Design review of the part built by this model. Coordinates are the model's own, in mm. A direction names the side the tool comes from. Give positions to 0.01 mm unless a question says otherwise; leave off trailing zeros. Loops run counter-clockwise (first coordinate to the right, second up) from the corner with the lowest first, then second, coordinate; pieces in that order, holes last. Notation, with made-up numbers: M 10.25,53 L 41.25,53 A10 ccw 41.25,68 Z; hole C 87.25,-13 d9. An arc over 180 degrees is marked long. Use CSV: the item, a comma, the result in double quotes.
from build123d import *

# Parameters (mm, degrees)
F0_R             = 14.605
F1_DEPTH         = 9.017
F2_R             = 6.35
F3_DEPTH         = 27.94
F4_R             = 5.334
F5_DEPTH         = 40.64
F6_R             = 8.255
F7_DEPTH         = 2.3
F8_R             = 5.06
F9_DEPTH         = 4.1
F11_D            = 3.1
F13_DEPTH        = 40.64
F13_COPIES_COUNT = 6
F14_R            = 0.508


# Not quite as in the source:
# - a pattern or mirror of a feature is missing from the dataset's text; its kind, count and spacing are read off the source's solid


with BuildPart() as f1:
    # F0 (on Top) → F1 (new body)
    with BuildSketch(Plane.XY):
        Circle(F0_R)
    extrude(amount=F1_DEPTH)

    # F2 (on face) → F3 (join)
    with BuildSketch(Plane.XY.offset(9.017)):
        Circle(F2_R)
    extrude(amount=F3_DEPTH)

    # F4 (on face) → F5 (join)
    with BuildSketch(Plane.XY.offset(36.957)):
        Circle(F4_R)
    extrude(amount=F5_DEPTH)

    # F6 (on face) → F7 (cut)
    with BuildSketch(Plane(origin=(0, 0, 0), x_dir=(1, 0, 0), z_dir=(0, 0, -1))):
        Circle(F6_R)
    extrude(amount=-F7_DEPTH, mode=Mode.SUBTRACT)

    # F8 (on face) → F9 (cut)
    with BuildSketch(Plane(origin=(0, 0, 0), x_dir=(1, 0, 0), z_dir=(0, 0, -1))):
        Circle(F8_R)
    extrude(amount=-F9_DEPTH, mode=Mode.SUBTRACT)

    # F11 (through all)
    with Locations(Plane.XY.offset(9.017)):
        with Locations((0, -10.05), (-10.05, 0), (0, 10.05), (10.05, 0)):
            Hole(F11_D / 2)

    # F12 (on face) → F13 (join, through all)
    with BuildSketch(Plane.XY.offset(77.597)):
        with BuildLine():
            Line((-1.27, -5.1806038258), (-1.27, -6.1957780109))
            ThreePointArc((-1.27, -6.1957780109), (0, -6.3246), (1.27, -6.1957780109))
            Line((1.27, -6.1957780109), (1.27, -5.1806038258))
            ThreePointArc((1.27, -5.1806038258), (0, -5.334), (-1.27, -5.1806038258))
        make_face()
    f13 = extrude(amount=-F13_DEPTH)

    # F13_copies: F13 ×6 about axis
    f13_copies_axis = Axis((0, 0, 0), (0, 0, 1))
    for i in range(1, F13_COPIES_COUNT):
        add(f13.rotate(f13_copies_axis, i * 360 / F13_COPIES_COUNT))

    # F14
    f14_edges = [f1.edges().sort_by_distance(p)[0] for p in [
        (1.27, -6.195778, 57.277),
        (1.27, -5.180604, 57.277),
        (-1.27, -6.195778, 57.277),
        (-1.27, -5.180604, 57.277),
        (3.851535, -3.690154, 57.277),
        (4.730701, -4.197741, 57.277),
        (6.000701, -1.998037, 57.277),
        (5.121535, -1.49045, 57.277),
        (5.121535, 1.49045, 57.277),
        (6.000701, 1.998037, 57.277),
        (4.730701, 4.197741, 57.277),
        (3.851535, 3.690154, 57.277),
        (1.27, 5.180604, 57.277),
        (1.27, 6.195778, 57.277),
        (-1.27, 6.195778, 57.277),
        (-1.27, 5.180604, 57.277),
        (-3.851535, 3.690154, 57.277),
        (-4.730701, 4.197741, 57.277),
        (-6.000701, 1.998037, 57.277),
        (-5.121535, 1.49045, 57.277),
        (-5.121535, -1.49045, 57.277),
        (-6.000701, -1.998037, 57.277),
        (-4.730701, -4.197741, 57.277),
        (-3.851535, -3.690154, 57.277),
    ]]
    fillet(f14_edges, radius=F14_R)


solid = f1.part
(1) Clearance check with flat-ended pins moving along their axes: P1, Ø6, axis at x = -8, z = 66.5, coming from the -Y side; P2, Ø10, axis at y = 2, z = 44, coming from the -X side; P3, Ø2, axis at y = 1, z = 66.5, coming from the +X side. State where each tip first meets the part, or that it passes through.
A:
P1,"y = -3.87"
P2,"x = -5.88"
P3,"x = 5.83"
(2) Machinability: for faces 4 (the cylindrical face through (-1.38, -6.2, 22.79)), 5 (the flat face through (0, 0, 4.1)), 6 (the cylindrical face through (5.483, 3.152, 57.561)), 7 (the cylindrical face through (-5.334, 0.016, 56.993)), 8 (the cylindrical face through (0.012, 6.325, 57.561)), which of the approach directions +Z, -Z, +X, -X, +Y, -Y give a long, thin tool a straight path to every point of the face, cutting with its end or side? Answer none if there is none.
A:
face 4,"+Z"
face 5,"-Z"
face 6,"+Z, +X, +Y"
face 7,"+Z, -X"
face 8,"+Z, +Y"
(3) We need section B-B on x = 0. State the section outline as (y, z) points (3 decimals), then the cut area to 3 significant figures.
A:
outline,"M -14.605,0 L -11.6,0 L -11.6,9.017 L -14.605,9.017 Z; M -8.5,0 L -8.255,0 L -8.255,2.3 L -5.06,2.3 L -5.06,4.1 L 5.06,4.1 L 5.06,2.3 L 8.255,2.3 L 8.255,0 L 8.5,0 L 8.5,9.017 L 6.35,9.017 L 6.35,36.957 L 6.325,36.957 L 6.325,77.597 L -6.325,77.597 L -6.325,36.957 L -6.35,36.957 L -6.35,9.017 L -8.5,9.017 Z; M 11.6,0 L 14.605,0 L 14.605,9.017 L 11.6,9.017 Z"
area,"1,020 mm²"
(4) We need section C-C on y = 10.05. State the section outline as (x, z) points, then the cut area to 3 significant figures.
A:
outline,"M -10.6,0 L -1.55,0 L -1.55,9.02 L -10.6,9.02 Z; M 1.55,0 L 10.6,0 L 10.6,9.02 L 1.55,9.02 Z"
area,"163 mm²"
(5) The part is to be moulded in two halves that separate along Y. For faces 1 (the cylindrical face through (-0.012, -6.325, 57.561)), 2 (the cylindrical face through (2.7, 4.6, 57)), 3 (the cylindrical face through (4.674, 1.938, 3.187)), say which applies: released by +Y, released by -Y, zero draft, split by the parting line, or undercut.
A:
face 1,"released by -Y"
face 2,"released by +Y"
face 3,"undercut"
(6) Wall thickness on line 1 along Y through (x, z) = (0, 3.75) (3 decimals); line 2 along Z through (x, y) = (-10, -5.25); line 3 along Z through (x, y) = (-1.75, -2.5): over which ranges is each line inside the solid? List them lowest first. Write a range as [from, to].
A:
line 1,"[-14.605, -11.6], [-8.5, -5.06], [5.06, 8.5], [11.6, 14.605]"
line 2,"[0, 9.02]"
line 3,"[4.1, 77.6]"
(7) We need section A-A on y = 0. State the section outline as (x, z) points (3 decimals).
A:
outline,"M -14.605,0 L -11.6,0 L -11.6,9.017 L -14.605,9.017 Z; M -8.5,0 L -8.255,0 L -8.255,2.3 L -5.06,2.3 L -5.06,4.1 L 5.06,4.1 L 5.06,2.3 L 8.255,2.3 L 8.255,0 L 8.5,0 L 8.5,9.017 L 6.35,9.017 L 6.35,36.957 L 5.334,36.957 L 5.334,77.597 L -5.334,77.597 L -5.334,36.957 L -6.35,36.957 L -6.35,9.017 L -8.5,9.017 Z; M 11.6,0 L 14.605,0 L 14.605,9.017 L 11.6,9.017 Z"
